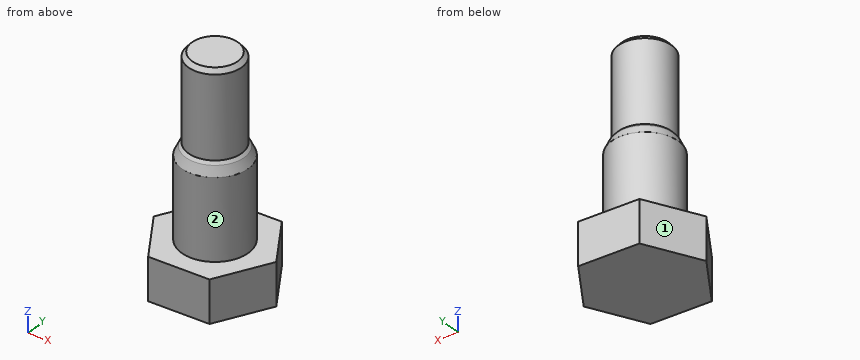
```python
from build123d import *

# Parameters (mm, degrees)
SKETCH_1_R      = 15
EXTRUDE_1_DEPTH = 1
EXTRUDE_2_DEPTH = 19
SKETCH_9_R      = 15
EXTRUDE_3_DEPTH = 36
SKETCH_11_R     = 15
EXTRUDE_6_DEPTH = 4
EXTRUDE_6_TAPER = 25
SKETCH_12_R     = 12
EXTRUDE_7_DEPTH = 38
SKETCH_13_R     = 13.134769367
EXTRUDE_8_DEPTH = 2
EXTRUDE_8_TAPER = 40
SKETCH_15_R     = 12
EXTRUDE_9_DEPTH = 2
EXTRUDE_9_TAPER = 40


with BuildPart() as part:
    # 草图1 → 拉伸1 (new body)
    with BuildSketch(Plane.XY):
        Circle(SKETCH_1_R)
    extrude(amount=EXTRUDE_1_DEPTH)

    # 草图2 → 拉伸2 (add)
    with BuildSketch(Plane.XY):
        Polygon((14.770690633, -22.071702054), (26.5, 1.755942292), (11.729309367, 23.827644346), (-14.770690633, 22.071702054), (-26.5, -1.755942292), (-11.729309367, -23.827644346), align=None)
    extrude(amount=EXTRUDE_2_DEPTH)

    # 草图9 → 拉伸3 (add)
    with BuildSketch(Plane.XY.offset(19)):
        Circle(SKETCH_9_R)
    extrude(amount=EXTRUDE_3_DEPTH)

    # 草图11 → 拉伸6 (add)
    with BuildSketch(Plane.XY.offset(55)):
        Circle(SKETCH_11_R)
    extrude(amount=EXTRUDE_6_DEPTH, taper=EXTRUDE_6_TAPER)

    # 草图12 → 拉伸7 (add)
    with BuildSketch(Plane.XY.offset(59)):
        Circle(SKETCH_12_R)
    extrude(amount=EXTRUDE_7_DEPTH)

    # 草图13 → 拉伸8 (add)
    with BuildSketch(Plane.XY.offset(59)):
        Circle(SKETCH_13_R)
    extrude(amount=EXTRUDE_8_DEPTH, taper=EXTRUDE_8_TAPER)

    # 草图15 → 拉伸9 (add)
    with BuildSketch(Plane.XY.offset(97)):
        Circle(SKETCH_15_R)
    extrude(amount=EXTRUDE_9_DEPTH, taper=EXTRUDE_9_TAPER)


solid = part.part
```
Could you check a few things on this model? Use its own coordinates, in mm. Face numbers are marked on the shaded views. A direction names the side the tool comes from. Round coordinates to 2 decimals unless told otherwise and drop trailing zeros. Write each loop counter-clockwise with the first axis right and the second up, starting at its lowest first coordinate (ties: lowest second). Pieces come first, ordered by that corner, then holes. Notation, with made-up numbers: M -9,33.25 L 14,33.25 A18 ccw 14,41.25 Z; hole C 24.5,-21 d5. An arc over 180 degrees is marked long. Answer in a Markdown table with one row per item. Add a question column.
Q1. Imagine slicing it at D-D (y = 19). Please give me the cut outline in (x, z), then the cut area to 3 significant figures.
Q2. Will these pins go through, and if not, where does the flat tip stop? pin 1 Ø2 at (x, z) = (-6.5, 85.5) entering from +Y; pin 2 Ø1.5 at (y, z) = (-3.5, 47) entering from -X; pin 3 Ø12 at (y, z) = (-4, 88.5) entering from +X.
Q3. If I drill on line 1 (Z direction, x = -10, y = 11.5); line 2 (Y direction, x = -0.5, z = 50); line 3 (X direction, y = 3, z = 77.5), over which ranges is the centre line in solid material (lowest first)? Write a range as from..to.
Q4. Imagine slicing it at C-C (z = 88.5). Please give me the cut outline in (x, y), then the cut area to 3 significant figures.
Q5. On a 3-axis mill with a long thin cutter (end or side, diameter ignored), from which of +Z, -Z, +X, -X, +Y, -Y can I reach the whole of each face in a straight line? I mean the marked faces 1 and 2. Say none if no direction works.
Q6. Imagine slicing it at B-B (y = 0). Please give me the cut outline in (x, z).
Q7. Imagine slicing it at A-A (x = 0). Please give me the cut outline in (y, z).
Values:
| question | item | result |
|---|---|---|
| 1 | outline | M -16.28,0 L 14.96,0 L 14.96,19 L -16.28,19 Z |
| 1 | area | 594 mm^2 |
| 2 | pin 1 | y = 10.67 |
| 2 | pin 2 | x = -14.75 |
| 2 | pin 3 | x = 12 |
| 3 | line 1 | 0..19 |
| 3 | line 2 | -14.99..14.99 |
| 3 | line 3 | -11.62..11.62 |
| 4 | outline | C 0,0 d24 |
| 4 | area | 452 mm^2 |
| 5 | face 1 | +Z, -Z, -X, +Y |
| 5 | face 2 | +Z |
| 6 | outline | M -25.64,0 L 25.64,0 L 25.64,19 L 15,19 L 15,55 L 13.13,59 L 12,60.35 L 12,97 L 10.32,99 L -10.32,99 L -12,97 L -12,60.35 L -13.13,59 L -15,55 L -15,19 L -25.64,19 Z |
| 7 | outline | M -23.05,0 L 23.05,0 L 23.05,19 L 15,19 L 15,55 L 13.13,59 L 12,60.35 L 12,97 L 10.32,99 L -10.32,99 L -12,97 L -12,60.35 L -13.13,59 L -15,55 L -15,19 L -23.05,19 Z |
